from build123d import *

# Parameters (mm, degrees)
SKETCH1_R                = 1.5
SKETCH1_W                = 26.67
SKETCH1_H                = 26.035
BOSS_EXTRUDE1_DEPTH      = 2.54
SKETCH3_W                = 1.27
SKETCH3_H                = 3.175
BOSS_EXTRUDE3_DEPTH      = 2.54
BOSS_EXTRUDE4_DEPTH      = 2.54
SKETCH5_W                = 1.27
SKETCH5_H                = 3.175
BOSS_EXTRUDE5_DEPTH      = 2.54
SKETCH7_W                = 1.27
SKETCH7_H                = 3.175
BOSS_EXTRUDE6_DEPTH      = 2.54
FILLET1_R                = 0.381
CUT_EXTRUDE2_REACH       = 16.605
SKETCH11_W               = 4.50557805
SKETCH11_H               = 5.61
SKETCH11_W_2             = 2.400870557
SKETCH11_H_2             = 3.07
SKETCH8_R                = 1.4224
BOSS_EXTRUDE7_DEPTH      = 1.905
BOSS_EXTRUDE7_DEPTH_BACK = 2.54
SKETCH10_R               = 1.6002
BOSS_EXTRUDE8_DEPTH      = 1.524
BOSS_EXTRUDE8_DEPTH_BACK = 2.54
FILLET2_R                = 0.635


with BuildPart() as part:
    # Sketch1 → Boss-Extrude1 (new body)
    with BuildSketch(Plane(origin=(0, 0, 0), x_dir=(1, 0, 0), z_dir=(0, 1, 0))):
        with BuildLine():
            Line((-10.16, -22.86), (-10.16, -5.715))
            Line((-10.16, -5.715), (-49.53, -5.715))
            Line((-49.53, -5.715), (-49.53, -3.175))
            Line((-49.53, -3.175), (-39.37, -3.175))
            Line((-39.37, -3.175), (-39.37, 22.86))
            Line((-39.37, 22.86), (-49.53, 22.86))
            Line((-49.53, 22.86), (-49.53, 25.4))
            Line((-49.53, 25.4), (-39.37, 25.4))
            Line((-39.37, 25.4), (-39.37, 30.443080793))
            Line((-39.37, 30.443080793), (-41.203087105, 33.618080793))
            ThreePointArc((-41.203087105, 33.618080793), (-38.1, 37.465), (-34.996912895, 33.618080793))
            Line((-34.996912895, 33.618080793), (-36.83, 30.443080793))
            Line((-36.83, 30.443080793), (-36.83, 25.4))
            Line((-36.83, 25.4), (-10.16, 25.4))
            Line((-10.16, 25.4), (-10.16, 30.48))
            Line((-10.16, 30.48), (-7.62, 30.48))
            Line((-7.62, 30.48), (-7.62, 25.4))
            Line((-7.62, 25.4), (-0.508, 25.4))
            Line((-0.508, 25.4), (-0.508, 22.86))
            Line((-0.508, 22.86), (-7.62, 22.86))
            Line((-7.62, 22.86), (-7.62, 1.27))
            Line((-7.62, 1.27), (-2.909935566, 1.27))
            ThreePointArc((-2.909935566, 1.27), (3.175, 0), (-2.909935566, -1.27))
            Line((-2.909935566, -1.27), (-7.62, -1.27))
            Line((-7.62, -1.27), (-7.62, -10.16))
            Line((-7.62, -10.16), (5.08, -10.16))
            Line((5.08, -10.16), (5.08, -12.7))
            Line((5.08, -12.7), (-7.62, -12.7))
            Line((-7.62, -12.7), (-7.62, -22.86))
            Line((-7.62, -22.86), (-10.16, -22.86))
        make_face()
        with Locations((-38.1, 34.29)):
            Circle(SKETCH1_R, mode=Mode.SUBTRACT)
        Circle(SKETCH1_R, mode=Mode.SUBTRACT)
        with Locations((-23.495, 9.8425)):
            Rectangle(SKETCH1_W, SKETCH1_H, mode=Mode.SUBTRACT)
    extrude(amount=BOSS_EXTRUDE1_DEPTH)

    # Sketch3 → Boss-Extrude3 (add)
    with BuildSketch(Plane.XY.offset(-22.86)):
        Polygon((-49.53, 2.54), (-49.53, 5.61), (-48.26, 5.61), (-46.99, 4.34), (-48.26, 4.34), (-48.26, 2.54), align=None)
        with Locations((-1.143, 4.1275)):
            Rectangle(SKETCH3_W, SKETCH3_H)
        Polygon((-16.51, 2.54), (-17.78, 2.54), (-17.78, 4.34), (-19.05, 4.34), (-17.78, 5.61), (-16.51, 5.61), align=None)
        with Locations((-13.4112, 4.1275)):
            Rectangle(SKETCH3_W, SKETCH3_H)
    extrude(amount=-BOSS_EXTRUDE3_DEPTH)

    # Sketch4 → Boss-Extrude4 (add)
    with BuildSketch(Plane.XY.offset(5.715)):
        Polygon((-17.78, 2.54), (-16.51, 2.54), (-16.51, 5.61), (-17.78, 5.61), (-19.05, 4.34), (-17.78, 4.34), align=None)
        Polygon((-49.53, 2.54), (-48.26, 2.54), (-48.26, 4.34), (-46.99, 4.34), (-48.26, 5.61), (-49.53, 5.61), align=None)
    extrude(amount=-BOSS_EXTRUDE4_DEPTH)

    # Sketch5 → Boss-Extrude5 (add)
    with BuildSketch(Plane(origin=(-7.62, 0, 0), x_dir=(0, 0, -1), z_dir=(1, 0, 0))):
        with Locations((6.477, 4.1275)):
            Rectangle(SKETCH5_W, SKETCH5_H)
        with Locations((29.845, 4.1275)):
            Rectangle(SKETCH5_W, SKETCH5_H)
    extrude(amount=-BOSS_EXTRUDE5_DEPTH)

    # Sketch7 → Boss-Extrude6 (add)
    with BuildSketch(Plane.XY.offset(12.7)):
        with Locations((4.445, 4.1275)):
            Rectangle(SKETCH7_W, SKETCH7_H)
    extrude(amount=-BOSS_EXTRUDE6_DEPTH)

    # Fillet1
    fillet1_edges = [part.edges().sort_by_distance(p)[0] for p in [
        (-46.99, 4.34, -24.13),
        (-19.05, 4.34, -24.13),
        (-46.99, 4.34, 4.445),
        (-19.05, 4.34, 4.445),
    ]]
    fillet(fillet1_edges, radius=FILLET1_R)

    # Sketch11 → Cut-Extrude2 (cut, up to next)
    with BuildSketch(Plane.XY.offset(-22.86), mode=Mode.PRIVATE) as cut_extrude2_sk1:
        with Locations((-47.277210975, 2.805)):
            Rectangle(SKETCH11_W, SKETCH11_H)
    cut_extrude2_tool1 = extrude(cut_extrude2_sk1.sketch, amount=-CUT_EXTRUDE2_REACH, mode=Mode.PRIVATE) & part.part
    add(cut_extrude2_tool1.solids().sort_by_distance((-47.277211, 2.805, -22.86))[0], mode=Mode.SUBTRACT)
    # Sketch11 → Cut-Extrude2 (cut, up to next)
    with BuildSketch(Plane.XY.offset(-22.86), mode=Mode.PRIVATE) as cut_extrude2_sk2:
        with Locations((-17.710435279, 4.075)):
            Rectangle(SKETCH11_W_2, SKETCH11_H_2)
    cut_extrude2_tool2 = extrude(cut_extrude2_sk2.sketch, amount=-CUT_EXTRUDE2_REACH, mode=Mode.PRIVATE) & part.part
    add(cut_extrude2_tool2.solids().sort_by_distance((-17.710435, 4.075, -22.86))[0], mode=Mode.SUBTRACT)

    # Sketch8 → Boss-Extrude7 (add, two sides)
    with BuildSketch(Plane(origin=(0, 2.54, 0), x_dir=(1, 0, 0), z_dir=(0, 1, 0))) as boss_extrude7_sk:
        with Locations((-44.52, 24.13)):
            Circle(SKETCH8_R)
        with Locations((-21.52, 24.13)):
            Circle(SKETCH8_R)
    extrude(amount=BOSS_EXTRUDE7_DEPTH)
    extrude(boss_extrude7_sk.sketch, amount=-BOSS_EXTRUDE7_DEPTH_BACK)

    # Sketch10 → Boss-Extrude8 (add, two sides)
    with BuildSketch(Plane(origin=(0, 2.54, 0), x_dir=(1, 0, 0), z_dir=(0, 1, 0))) as boss_extrude8_sk:
        with Locations((-8.89, -7.7216)):
            Circle(SKETCH10_R)
        with Locations((-8.89, -22.86)):
            Circle(SKETCH10_R)
    extrude(amount=BOSS_EXTRUDE8_DEPTH)
    extrude(boss_extrude8_sk.sketch, amount=-BOSS_EXTRUDE8_DEPTH_BACK)

    # Fillet2
    fillet2_edges = [part.edges().sort_by_distance(p)[0] for p in [
        (-45.9424, 4.445, -24.13),
        (-22.9424, 4.445, -24.13),
        (-10.4902, 4.064, 7.7216),
        (-10.4902, 4.064, 22.86),
    ]]
    fillet(fillet2_edges, radius=FILLET2_R)


solid = part.part
Work out the finished part from the listing and answer in its coordinate system (mm). A direction names the side the tool comes from. Coordinates: 2 decimals unless noted, no trailing zeros. Write each loop counter-clockwise with the first axis right and the second up, starting at its lowest first coordinate (ties: lowest second). Pieces come first, ordered by that corner, then holes. Notation, with made-up numbers: M -27,27 L 10,27 A19 cw 10,62 Z; hole C 16,70 d2. An arc over 180 degrees is marked long. Use one line per item in the form item = value. Start each with the question number.
1. Each of these flat-tipped pins is pushed along its axis until it touches: P1, Ø1.7, axis at x = -14.5, y = 2.5, coming from the +Z side (3 decimals); P2, Ø3, axis at x = -1.5, y = 3, coming from the -Z side; P3, Ø3, axis at y = 3.5, z = 11.5, coming from the -X side; P4, Ø1.5, axis at x = -38, z = 2.5, coming from the -Y side. Where does it stop, or does it pass through?
2. The part is cut by section D-D (x = -8.89). Give the vertices of the cut face in (y, z) (3 decimals).
3. The part is cut by section B-B (z = -34.29). Give the vertices of the cut face in (x, y) (3 decimals).
4. The part is cut by section A-A (x = -25.5). Give the vertices of the cut face in (y, z) (3 decimals).
5. Straight lines are drawn through the part: probe 1 along Z at (x, y) = (0, 1.85) (3 decimals); probe 2 along X at (y, z) = (0.7, 0) (3 decimals); probe 3 along Z at (x, y) = (-20, 0.45) (3 decimals). For each, find the intervals that lie inside material, in ascending order. Write a range as from..to.
6. A tool of negligible diameter and unlimited length cuts with its end or side. For faces 3 (the face through (-7.62, 2, -28)), 4 (the face through (-7.62, 1, 4)), 5 (the face through (-9, 4.064, 23)), 6 (the face through (-45, 4.445, -24)), 7 (the face through (-1, 2, 10.16)), from which of +Z, -Z, +X, -X, +Y, -Y can it reach the whole face along a straight path? Write none if from no direction.
7. The mould has two halves that part along Z. Classify faces 1 (the face through (-9, 5.715, -6)), 2 (the face through (-36.83, 1, -10)): released by +Z, released by -Z, zero draft, split by the parting line, or undercut.
8. The part is cut by section C-C (z = -24.13). Give the vertices of the cut face in (x, y) (3 decimals), plus the area to 3 significant figures.
Evaluation:
q1.P1 = 5.715
q1.P2 = -25.4
q1.P3 = -10.16
q1.P4 = 0
q2.outline = M 0,-30.48 L 5.715,-30.48 L 5.715,-29.21 L 2.54,-29.21 L 2.54,-7.112 L 5.715,-7.112 L 5.715,-5.842 L 2.54,-5.842 L 2.54,6.121 L 3.429,6.121 A0.635 ccw 4.064,6.756 L 4.064,8.687 A0.635 ccw 3.429,9.322 L 2.54,9.322 L 2.54,21.26 L 3.429,21.26 A0.635 ccw 4.064,21.895 L 4.064,23.825 A0.635 ccw 3.429,24.46 L 0,24.46 Z
q3.outline = M -41.275,0 L -39.6,0 L -39.6,2.54 L -41.275,2.54 Z; M -36.6,0 L -34.925,0 L -34.925,2.54 L -36.6,2.54 Z
q4.outline = M 0,-25.4 L 2.54,-25.4 L 2.54,-22.86 L 0,-22.86 Z; M 0,3.175 L 2.54,3.175 L 2.54,5.715 L 0,5.715 Z
q5.probe_1 = -3.175..-1.5, 1.5..3.175, 10.16..12.7
q5.probe_2 = -39.37..-36.83, -10.16..-1.5, 1.5..3.175
q5.probe_3 = -25.4..-22.86, 3.175..5.715
q6.face_3 = -Z, +X, +Y, -Y
q6.face_4 = +Y, -Y
q6.face_5 = +Z, +X, -X, +Y
q6.face_6 = +Z, -Z, -X, +Y
q6.face_7 = +X, +Y, -Y
q7.face_1 = zero draft
q7.face_2 = undercut
q8.outline = M -45.942,0 L -0.508,0 L -0.508,5.715 L -1.778,5.715 L -1.778,2.54 L -12.776,2.54 L -12.776,5.715 L -14.046,5.715 L -14.046,2.54 L -20.098,2.54 L -20.098,3.81 A0.635 ccw -20.733,4.445 L -22.307,4.445 A0.635 ccw -22.942,3.81 L -22.942,2.54 L -43.098,2.54 L -43.098,3.81 A0.635 ccw -43.733,4.445 L -45.307,4.445 A0.635 ccw -45.942,3.81 Z
q8.area = 134 mm^2
